Geometry: final body of the model. Coordinates: model frame, mm. A direction names the side the tool comes from. Give positions to 0.01 mm unless a question says otherwise; leave off trailing zeros. Order: outer loops, then holes, each group sorted by start corner. A loop starts at its lowest first (then second) coordinate and runs counter-clockwise, first axis right, second up. Notation, with made-up numbers: (15, 46.25) -> (69, 46.25) arc R10 ccw to (69, 62.25) -> close; hole circle Ø4 at (-1, 37). An arc over 180 degrees is marked (long way). One line per question, with ' | ' between items.
from build123d import *

# Parameters (mm, degrees)
PROFILE_DEPTH = 10.25
POCKET_DEPTH  = 19.5
HOLES_R       = 2
HOLE_DEPTH    = 1


with BuildPart() as part:
    # ProfileS → Profile (new, symmetric)
    with BuildSketch(Plane.XY):
        with BuildLine():
            Line((-3, 3.2), (3, 3.2))
            ThreePointArc((3, 3.2), (6.2, 0), (3, -3.2))
            Line((3, -3.2), (-3, -3.2))
            ThreePointArc((-3, -3.2), (-6.2, 0), (-3, 3.2))
        make_face()
    extrude(amount=PROFILE_DEPTH, both=True)

    # PocketS → Pocket (cut)
    with BuildSketch(Plane.XY.offset(10.25)):
        with BuildLine():
            Line((-3, -2.7), (3, -2.7))
            ThreePointArc((3, -2.7), (5.7, 0), (3, 2.7))
            Line((3, 2.7), (-3, 2.7))
            ThreePointArc((-3, 2.7), (-5.7, 0), (-3, -2.7))
        make_face()
    extrude(amount=-POCKET_DEPTH, mode=Mode.SUBTRACT)

    # HoleS → Hole (cut)
    with BuildSketch(Plane(origin=(0, 0, -10.25), x_dir=(-1, 0, 0), z_dir=(0, 0, -1))):
        Circle(HOLES_R)
    extrude(amount=-HOLE_DEPTH, mode=Mode.SUBTRACT)


solid = part.part
1) Section B-B on z = 4. Return loops of the section in (x, y).
Check result:
outline: (-3, -3.2) -> (3, -3.2) arc R3.2 ccw to (3, 3.2) -> (-3, 3.2) arc R3.2 ccw to start; hole (-3, -2.7) -> (3, -2.7) arc R2.7 ccw to (3, 2.7) -> (-3, 2.7) arc R2.7 ccw to start
2) Section A-A on x = 0. Return loops of the section in (y, z), plus the area to 3 significant figures.
Check result:
outline: (-3.2, -10.25) -> (-2, -10.25) -> (-2, -9.25) -> (-2.7, -9.25) -> (-2.7, 10.25) -> (-3.2, 10.25) -> close; (2, -10.25) -> (3.2, -10.25) -> (3.2, 10.25) -> (2.7, 10.25) -> (2.7, -9.25) -> (2, -9.25) -> close | area: 21.9 mm^2
3) Section C-C on y = -0.25. Return loops of the section in (x, z).
Check result:
outline: (-6.19, -10.25) -> (-1.98, -10.25) -> (-1.98, -9.25) -> (-5.69, -9.25) -> (-5.69, 10.25) -> (-6.19, 10.25) -> close; (1.98, -10.25) -> (6.19, -10.25) -> (6.19, 10.25) -> (5.69, 10.25) -> (5.69, -9.25) -> (1.98, -9.25) -> close
4) Pull-direction query (Y, two-part tool) for faces 1 (the flat face through (0, 3.2, 0)), 2 (the cylindrical face through (5.7, -0.1, 0.6)), 3 (the cylindrical face through (-6.2, -0.1, 0.1)); classes: +Y half, -Y half, draft (parallel to the pull), parting line (faces both ways), or undercut.
Check result:
face 1: +Y half | face 2: undercut | face 3: parting line
5) Set-up query: faces 4 (the cylindrical face through (-5.7, 0.1, 0.6)), 5 (the cylindrical face through (6.2, 0.1, 0.1)). Return all of +Z, -Z, +X, -X, +Y, -Y with unobstructed straight access to the full face (end or side cutting, diameter ignored); none if empty.
Check result:
face 4: +Z | face 5: +Z, -Z, +X
6) Section D-D on x = 2.25. Return loops of the section in (y, z).
Check result:
outline: (-3.2, -10.25) -> (3.2, -10.25) -> (3.2, 10.25) -> (2.7, 10.25) -> (2.7, -9.25) -> (-2.7, -9.25) -> (-2.7, 10.25) -> (-3.2, 10.25) -> close
7) Material intervals for probe 1 along Y at (x, z) = (0, -9.5); probe 2 along Y at (x, z) = (-2.75, 6.5); probe 3 along X at (y, z) = (0, 8.75), sorted ascending. Write a range as from..to.
Check result:
probe 1: y = -3.2..-2, 2..3.2 | probe 2: y = -3.2..-2.7, 2.7..3.2 | probe 3: x = -6.2..-5.7, 5.7..6.2
